Can you work these out from the drawing? Everything is in mm from the part's minimum corner. Round coordinates to 2 decimals unless told otherwise and drop trailing zeros. Write each loop counter-clockwise with the first axis right and the second up, starting at its lowest first coordinate (ties: lowest second). Pieces come first, ordered by that corner, then holes.
Q1. Please list where these lines run through material, in increasing order: line 1 along X through (y, z) = (0.75, 43.5); line 2 along Z through (x, y) = (109, 0.75).
Q2. If we section it at A-A (z = 45): Please give me the cut outline in (x, y).
Q3. I'm going to push flat-ended pins straight in: pin 1 Ø1.9 at (y, z) = (1.5, 70.5) entering from -X; pin 2 Ø1 at (x, y) = (161.5, 2.5) entering from -Z; pin 3 Ø3 at (y, z) = (2, 3.5) entering from +X. Where does each tip first touch, or does it pass through?
Q4. If we section it at B-B (x = 65): Please give me the cut outline in (y, z).
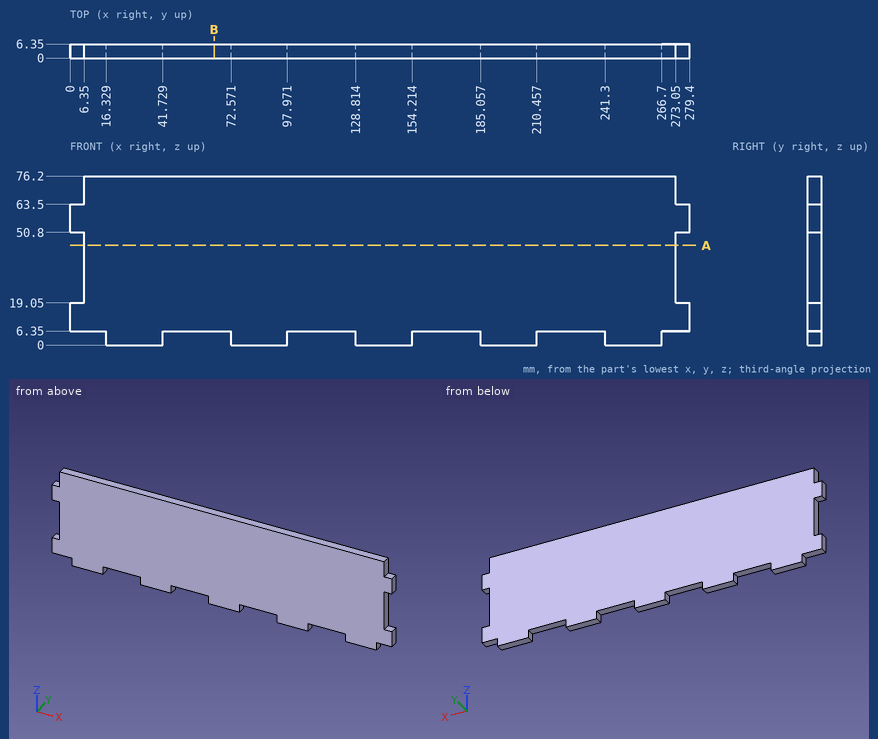
A:
1. line 1: x = 6.35 to 273.05
1. line 2: z = 6.35 to 76.2
2. outline: (6.35, 0) - (273.05, 0) - (273.05, 6.35) - (6.35, 6.35) - close
3. pin 1: stops at x = 6.35
3. pin 2: stops at z = 6.35
3. pin 3: stops at x = 266.7
4. outline: (0, 6.35) - (6.35, 6.35) - (6.35, 76.2) - (0, 76.2) - close
